Geometry check sheet. Reference: drawing and pictorial views, mm from the part's lowest x, y, z. Coordinates: 2 decimals unless noted, no trailing zeros. Loops run counter-clockwise (first coordinate to the right, second up) from the corner with the lowest first, then second, coordinate; pieces in that order, holes last. Notation, with made-up numbers: (-13, -12) -> (32, -12) arc R25 cw to (32, 14) -> close; hole circle Ø8 at (-29, 71). An arc over 180 degrees is marked (long way). Use CSV: the item, a comma, the result in double quotes.
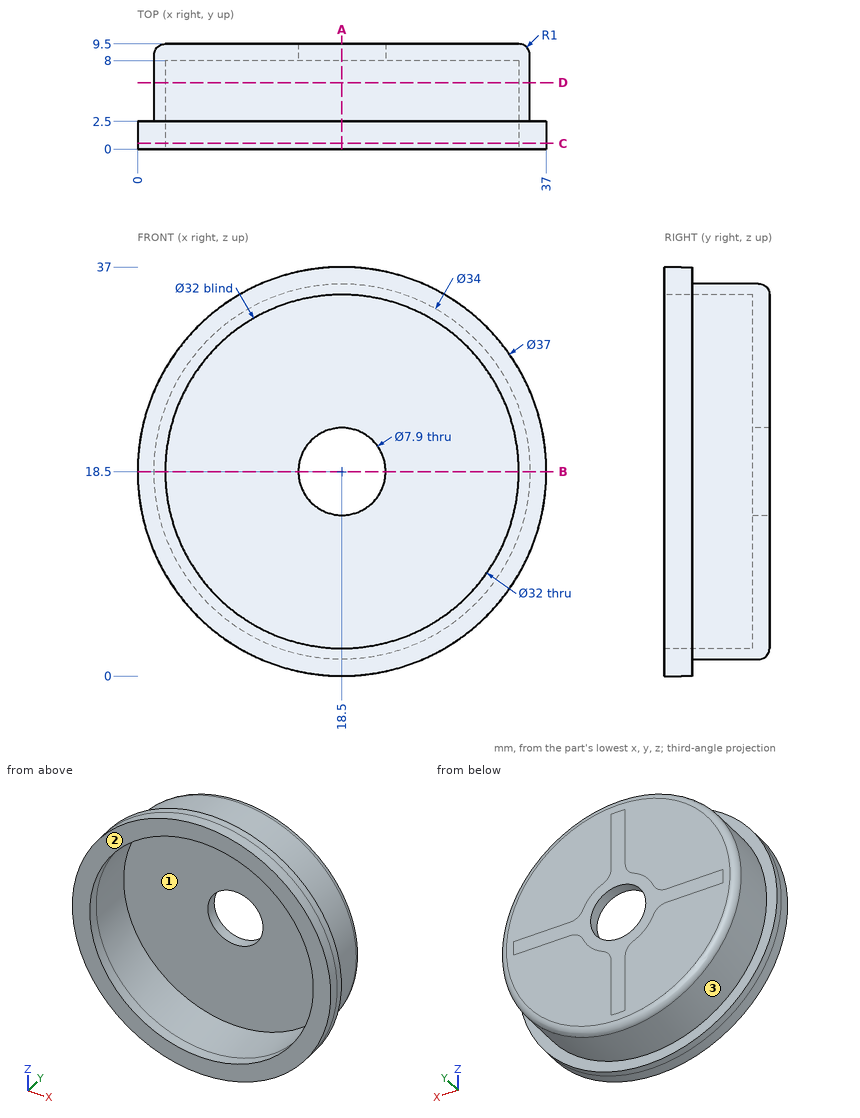
1) Draft check along Z on the marked faces 1, 2 and 3. Enter one of: released by +Z, released by -Z, zero draft, split by the parting line, or undercut.
Answer below:
face 1,"undercut"
face 2,"zero draft"
face 3,"split by the parting line"
2) Thickness scan on line 1 along X through (y, z) = (4.5, 18.5); line 2 along X through (y, z) = (8.55, 18.5); line 3 along Z through (x, y) = (19, 3.75). Record the ranges inside material, lowest first. Write a range as from..to.
Answer below:
line 1,"x = 1.5..2.5, 34.5..35.5"
line 2,"x = 1.5..14.55, 22.45..35.5"
line 3,"z = 1.51..2.51, 34.49..35.49"
3) Cross-section at C-C on y = 0.5. Record the boundary of the cut face in (x, z), and give its area (3 significant figures).
Answer below:
outline,"circle Ø37 at (18.5, 18.5); hole circle Ø32 at (18.5, 18.5)"
area,"271 mm²"
4) Cross-section at A-A on x = 18.5. Record the boundary of the cut face in (y, z), and give its area (3 significant figures).
Answer below:
outline,"(0, 0) -> (2.5, 0) -> (2.5, 1.5) -> (8.5, 1.5) arc R1 ccw to (9.5, 2.5) -> (9.5, 14.55) -> (8, 14.55) -> (8, 2.5) -> (0, 2.5) -> close; (0, 34.5) -> (8, 34.5) -> (8, 22.45) -> (9.5, 22.45) -> (9.5, 34.5) arc R1 ccw to (8.5, 35.5) -> (2.5, 35.5) -> (2.5, 37) -> (0, 37) -> close"
area,"62.2 mm²"
5) Cross-section at D-D on y = 6. Record the boundary of the cut face in (x, z).
Answer below:
outline,"circle Ø34 at (18.5, 18.5); hole circle Ø32 at (18.5, 18.5)"
6) Go/stop test with flat-tipped pins: pin 1 Ø1 at (y, z) = (1.5, 26) entering from +X; pin 2 Ø6 at (x, z) = (24.5, 29.5) entering from -Y; pin 3 Ø1 at (x, y) = (8.5, 8) entering from +Z. Record where each tip stops, or that it passes through.
Answer below:
pin 1,"stops at x = 35.62"
pin 2,"stops at y = 8"
pin 3,"stops at z = 32.6"
7) Cross-section at B-B on z = 18.5. Record the boundary of the cut face in (x, y), and give its area (3 significant figures).
Answer below:
outline,"(0, 0) -> (2.5, 0) -> (2.5, 8) -> (14.55, 8) -> (14.55, 9.5) -> (2.5, 9.5) arc R1 ccw to (1.5, 8.5) -> (1.5, 2.5) -> (0, 2.5) -> close; (22.45, 8) -> (34.5, 8) -> (34.5, 0) -> (37, 0) -> (37, 2.5) -> (35.5, 2.5) -> (35.5, 8.5) arc R1 ccw to (34.5, 9.5) -> (22.45, 9.5) -> close"
area,"62.2 mm²"
